The model under review builds one solid part; all positions refer to its coordinate system, in mm. Face numbers are marked on the shaded views. A direction names the side the tool comes from. Coordinates: 2 decimals unless noted, no trailing zeros. Write each loop counter-clockwise with the first axis right and the second up, starting at its lowest first coordinate (ties: lowest second). Pieces come first, ordered by that corner, then holes. Notation, with made-up numbers: (20, 73.25) - (34, 73.25) arc R20 cw to (34, 95.25) - close; hole circle Ø8 at (57.25, -4.5). An arc over 180 degrees is marked (long way). Put each result on its own line as item: value.
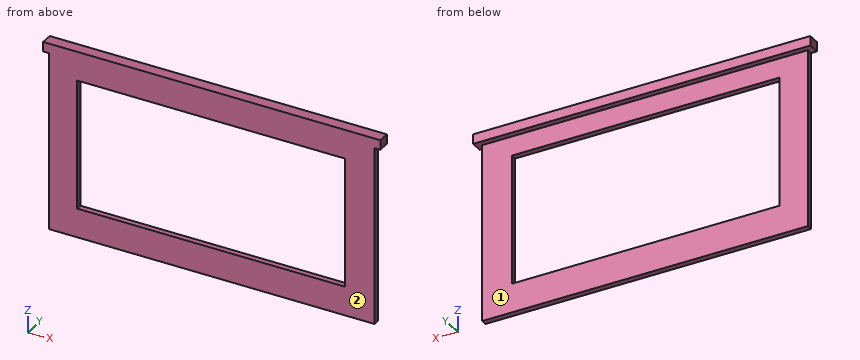
from build123d import *

# Parameters (mm, degrees)
SKETCH1_W           = 169
SKETCH1_H           = 6
BOSS_EXTRUDE1_DEPTH = 5
SKETCH2_W           = 169
SKETCH2_H           = 3
BOSS_EXTRUDE2_DEPTH = 92
SKETCH3_W           = 5
SKETCH3_H           = 6
BOSS_EXTRUDE3_DEPTH = 3
SKETCH4_W           = 5
SKETCH4_H           = 6
BOSS_EXTRUDE4_DEPTH = 3
SKETCH8_W           = 139
SKETCH8_H           = 67
CUT_EXTRUDE2_DEPTH  = 3


with BuildPart() as part:
    # Sketch1 → Boss-Extrude1 (new body)
    with BuildSketch(Plane.XY):
        Rectangle(SKETCH1_W, SKETCH1_H)
    extrude(amount=-BOSS_EXTRUDE1_DEPTH)

    # Sketch2 → Boss-Extrude2 (add)
    with BuildSketch(Plane(origin=(0, 0, -5), x_dir=(-1, 0, 0), z_dir=(0, 0, -1))):
        with Locations((0, -1.5)):
            Rectangle(SKETCH2_W, SKETCH2_H)
    extrude(amount=BOSS_EXTRUDE2_DEPTH)

    # Sketch3 → Boss-Extrude3 (add)
    with BuildSketch(Plane(origin=(84.5, 0, 0), x_dir=(0, 0, -1), z_dir=(1, 0, 0))):
        with Locations((2.5, 0)):
            Rectangle(SKETCH3_W, SKETCH3_H)
    extrude(amount=BOSS_EXTRUDE3_DEPTH)

    # Sketch4 → Boss-Extrude4 (add)
    with BuildSketch(Plane.ZY.offset(84.5)):
        with Locations((-2.5, 0)):
            Rectangle(SKETCH4_W, SKETCH4_H)
    extrude(amount=BOSS_EXTRUDE4_DEPTH)

    # Sketch8 → Cut-Extrude2 (cut)
    with BuildSketch(Plane(origin=(0, 0, 0), x_dir=(1, 0, 0), z_dir=(0, 1, 0))):
        with Locations((-0.408697147, 48.504527108)):
            Rectangle(SKETCH8_W, SKETCH8_H)
    extrude(amount=-CUT_EXTRUDE2_DEPTH, mode=Mode.SUBTRACT)


solid = part.part
1. Consider section D-D on z = -10. State the section outline as (x, y) points.
Determined:
outline: (-84.5, -3) - (84.5, -3) - (84.5, 0) - (-84.5, 0) - close
2. Consider section A-A on x = 6.5. State the section outline as (y, z) points.
Determined:
outline: (-3, -97) - (0, -97) - (0, -82) - (-3, -82) - close; (-3, -15) - (0, -15) - (0, -5) - (3, -5) - (3, 0) - (-3, 0) - close
3. Consider section B-B on z = -46.5. State the section outline as (x, y) points, plus the area to 3 significant figures.
Determined:
outline: (-84.5, -3) - (-69.91, -3) - (-69.91, 0) - (-84.5, 0) - close; (69.09, -3) - (84.5, -3) - (84.5, 0) - (69.09, 0) - close
area: 90.0 mm^2
4. For pin 1 Ø2.5 at (y, z) = (-1.5, -73) entering from +X; pin 2 Ø3.5 at (y, z) = (-1, -35) entering from -X; pin 3 Ø2 at (x, y) = (-44, 2) entering from -Z, all flat-tipped, find the tip position at first contact; note any pin that passes through.
Determined:
pin 1: stops at x = 84.5
pin 2: stops at x = -84.5
pin 3: stops at z = -5
5. Consider section C-C on y = -2. State the section outline as (x, z) points.
Determined:
outline: (-87.5, -5) - (-84.5, -5) - (-84.5, -97) - (84.5, -97) - (84.5, -5) - (87.5, -5) - (87.5, 0) - (-87.5, 0) - close; hole (-69.91, -82) - (69.09, -82) - (69.09, -15) - (-69.91, -15) - close
6. To check wall thickness, follow probe 1 along X at (y, z) = (-0.55, -46); probe 2 along Z at (x, y) = (-31.5, -0.2); probe 3 along Z at (x, y) = (-62, 1.65). State the ranges of each line that lie inside material, in increasing order.
Determined:
probe 1: x = -84.5 to -69.91, 69.09 to 84.5
probe 2: z = -97 to -82, -15 to 0
probe 3: z = -5 to 0
7. Machinability: for the marked faces 1 and 2, which of the approach directions +Z, -Z, +X, -X, +Y, -Y give a long, thin tool a straight path to every point of the face, cutting with its end or side? Answer none if there is none.
Determined:
face 1: -Z, +X, -X, +Y
face 2: +Z, -Z, +X, -X, -Y
